Verification items for the finished model (mm, model axes). Give positions to 0.01 mm unless a question says otherwise; leave off trailing zeros. Write each loop counter-clockwise with the first axis right and the second up, starting at its lowest first coordinate (ties: lowest second). Pieces come first, ordered by that corner, then holes. Notation, with made-up numbers: (-34.75, 13.5) -> (3.25, 13.5) arc R24 ccw to (3.25, 51.5) -> close; hole circle Ø1 at (35.5, -31). An arc over 180 degrees is marked (long way). Write item = value, one per line.
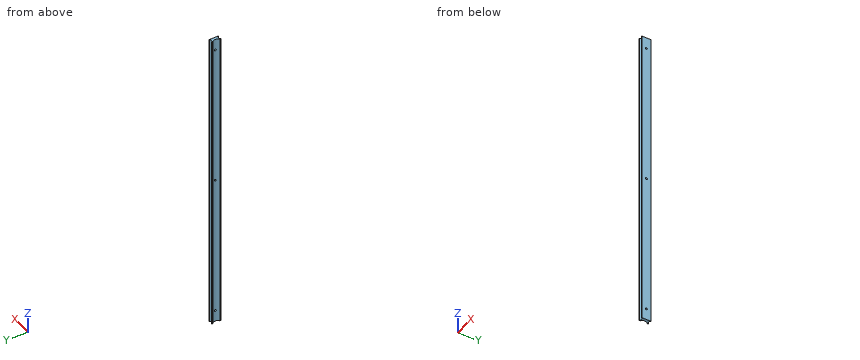
from build123d import *

# Parameters (mm, degrees)
SKETCH_1_W          = 5.6
SKETCH_1_H          = 12
EXTRUDE_1_DEPTH     = 200
SKETCH_2_R          = 2.5
CUT_EXTRUDE_1_DEPTH = 230
SKETCH_3_R          = 5.5
CUT_EXTRUDE_2_DEPTH = 690
HOLE_WIZARD_M3_1_D  = 2.5


with BuildPart() as part:
    # 草图1 → 凸台-拉伸1 (new, symmetric)
    with BuildSketch(Plane.XY):
        Rectangle(SKETCH_1_W, SKETCH_1_H)
    extrude(amount=EXTRUDE_1_DEPTH, both=True)

    # 草图2 → 切除-拉伸1 (cut, symmetric)
    with BuildSketch(Plane.XY):
        with Locations((0, 7)):
            Circle(SKETCH_2_R)
    cut_extrude_1 = extrude(amount=CUT_EXTRUDE_1_DEPTH, both=True, mode=Mode.SUBTRACT)

    # 镜向1: 切除-拉伸1 across plane
    add(cut_extrude_1.mirror(Plane.ZX), mode=Mode.SUBTRACT)

    # 草图3 → 切除-拉伸2 (cut, symmetric)
    with BuildSketch(Plane.XY.offset(200)):
        with Locations((-6, 0)):
            Circle(SKETCH_3_R)
    extrude(amount=CUT_EXTRUDE_2_DEPTH, both=True, mode=Mode.SUBTRACT)

    # M3 螺纹孔1 (through all)
    with Locations(Plane(origin=(2.8, 0, 0), x_dir=(0, 0, -1), z_dir=(1, 0, 0))):
        with Locations((-185, 0), (0, 0), (185, 0)):
            Hole(HOLE_WIZARD_M3_1_D / 2)


solid = part.part
Item 1: Material ranges on line 1 (Z direction, x = 0.1, y = 0); line 2 (Z direction, x = 2.55, y = 1); line 3 (Y direction, x = 0.55, z = -185), recorded low to high.
Response values:
line_1 = -200 to -186.25, -183.75 to -1.25, 1.25 to 183.75, 186.25 to 200
line_2 = -200 to -185.75, -184.25 to -0.75, 0.75 to 184.25, 185.75 to 200
line_3 = -4.56 to -1.25, 1.25 to 4.56
Item 2: Sectioned sample at B-B on x = 0.85. Record the cut outline in (y, z), then the cut area to 3 significant figures.
Response values:
outline = (-4.65, -200) -> (4.65, -200) -> (4.65, 200) -> (-4.65, 200) -> close; hole circle Ø2.5 at (0, -185); hole circle Ø2.5 at (0, 0); hole circle Ø2.5 at (0, 185)
area = 3,700 mm^2
Item 3: Sectioned sample at A-A on z = 6. Record the cut outline in (x, y).
Response values:
outline = (-2.8, -6) -> (-2.29, -6) arc R2.5 cw to (2.29, -6) -> (2.8, -6) -> (2.8, 6) -> (2.29, 6) arc R2.5 cw to (-2.29, 6) -> (-2.8, 6) -> (-2.8, 4.47) arc R5.5 cw to (-2.8, -4.47) -> close
Item 4: Go/stop test with flat-tipped pins: P1, Ø1.5, axis at y = -1, z = 146.5, coming from the -X side; P2, Ø3, axis at y = 0, z = 185, coming from the -X side; P3, Ø2, axis at y = 0, z = 0, coming from the +X side; P4, Ø1.5, axis at y = 2, z = -89, coming from the -X side. Record where each tip stops, or that it passes through.
Response values:
P1 = -0.79
P2 = -0.71
P3 = through
P4 = -1.24
